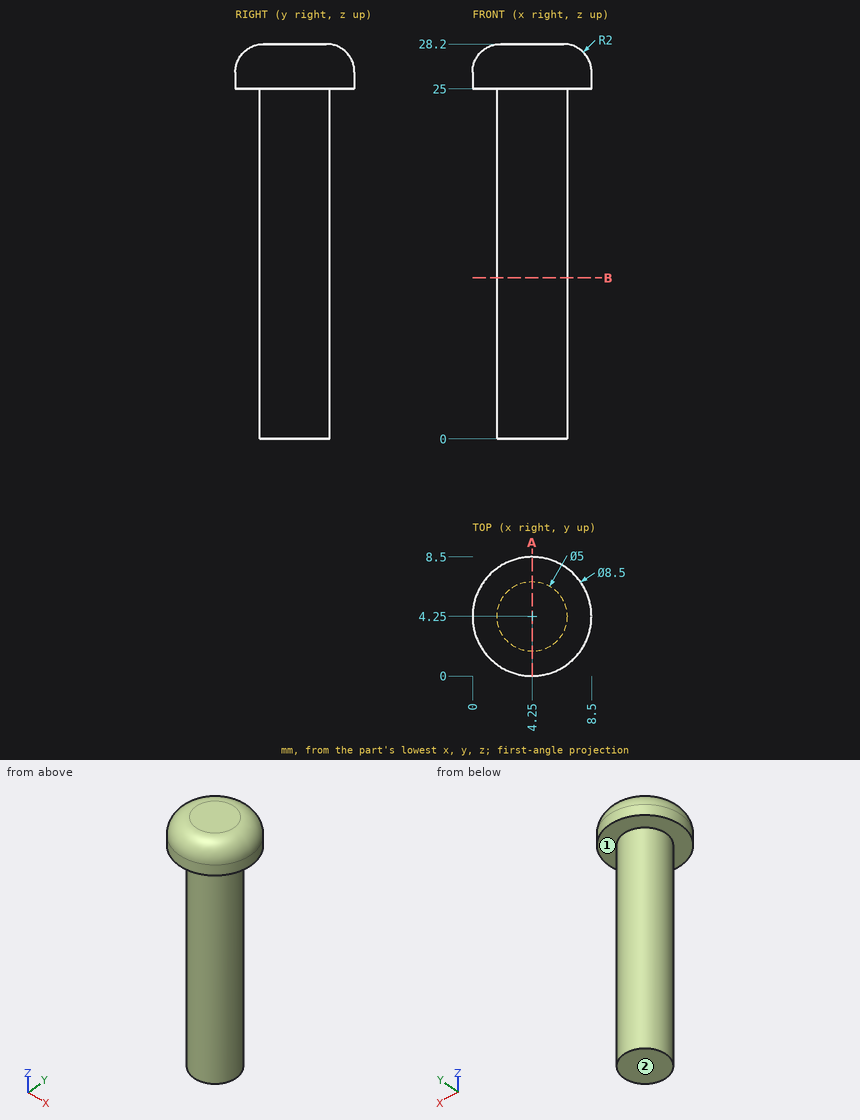
Study the drawing (mm; zero at the part's minimum x, y, z) and answer. A direction names the side the tool comes from. Coordinates: 2 decimals unless noted, no trailing zeros. Write each loop counter-clockwise with the first axis right and the second up, starting at its lowest first coordinate (ties: lowest second). Pieces come first, ordered by that corner, then holes.
Q1. A cutting plane is placed at A-A, the plane x = 4.25. Give the vertices of the cut face in (y, z), then the cut area to 3 significant figures.
Q2. Each of these flat-tipped pins is pushed along its axis until it touches: pin 1 Ø5 at (x, z) = (4, 17) entering from -Y; pin 2 Ø1.5 at (y, z) = (3, 20) entering from -X; pin 3 Ø1.5 at (y, z) = (2, 5) entering from +X. Where does it stop, or does it pass through?
Q3. Find the intervals of material crossed by line 1 (Y direction, x = 4.25, z = 16.25); line 2 (Z direction, x = 6, y = 1); line 3 (Z direction, x = 1, y = 3), in increasing order.
Q4. A cutting plane is placed at B-B, the plane z = 11.5. Give the vertices of the cut face in (x, y), then the cut area to 3 significant figures.
Q5. Which of the six approach directions +Z, -Z, +X, -X, +Y, -Y give full straight-line access (tool end or side, diameter ignored) to the marked faces 1 and 2?
Findings below:
1. outline: (0, 25) - (1.75, 25) - (1.75, 0) - (6.75, 0) - (6.75, 25) - (8.5, 25) - (8.5, 26.2) arc R2 ccw to (6.5, 28.2) - (2, 28.2) arc R2 ccw to (0, 26.2) - close
1. area: 150 mm2
2. pin 1: stops at y = 1.75
2. pin 2: stops at x = 1.8
2. pin 3: stops at x = 6.25
3. line 1: y = 1.75 to 6.75
3. line 2: z = 25 to 27.59
3. line 3: z = 25 to 27.78
4. outline: circle Ø5 at (4.25, 4.25)
4. area: 19.6 mm2
5. face 1: -Z
5. face 2: -Z, +X, -X, +Y, -Y
